Build history of the part. All positions in model axes, mm. A direction names the side the tool comes from. Round coordinates to 2 decimals unless told otherwise and drop trailing zeros. Write each loop counter-clockwise with the first axis right and the second up, starting at its lowest first coordinate (ties: lowest second). Pieces come first, ordered by that corner, then holes. Notation, with made-up numbers: (-1.5, -7) -> (11.5, -7) arc R18 ccw to (11.5, -1) -> close; hole circle Ø2 at (53, -9.5). An arc over 180 degrees is marked (long way). Answer as CSV lines item,"result".
from build123d import *

# Parameters (mm, degrees)
SKETCH_W        = 200
SKETCH_H        = 120
PAD_DEPTH       = 60
SKETCH002_R     = 16
POCKET001_DEPTH = 5
POCKET_DEPTH    = 58
SKETCH004_R     = 1.65
HOLE_DEPTH      = 4
SKETCH005_R     = 4
POCKET002_DEPTH = 3
SKETCH006_R     = 4.4
HOLE001_DEPTH   = 22.356213
HOLE001_TIPS_R  = 4.4
SKETCH007_R     = 2.5
HOLE002_DEPTH   = 25
FILLET_R        = 4.5
FILLET001_R     = 4.5
SKETCH008_R     = 1.65
HOLE003_DEPTH   = 9.00858
HOLE003_TIPS_R  = 1.65


with BuildPart() as part:
    # Sketch → Pad (new body)
    with BuildSketch(Plane.XY):
        Rectangle(SKETCH_W, SKETCH_H)
    extrude(amount=PAD_DEPTH)

    # Sketch002 (on Face3 of Pad) → Pocket001 (cut)
    with BuildSketch(Plane.XZ.offset(60)):
        with Locations((-53.5, 31)):
            Circle(SKETCH002_R)
        with Locations((-12, 31)):
            Circle(SKETCH002_R)
        with Locations((29.5, 31)):
            Circle(SKETCH002_R)
        with Locations((71, 31)):
            Circle(SKETCH002_R)
    extrude(amount=-POCKET001_DEPTH, mode=Mode.SUBTRACT)

    # Sketch003 (on Face6 of Pad) → Pocket (cut)
    with BuildSketch(Plane.XY.offset(60)):
        Polygon((-87.5, 57), (87.5, 57), (87.5, 38.5), (95.5, 38.5), (95.5, -38.5), (87.5, -38.5), (87.5, -57), (-87.5, -57), (-87.5, -38.5), (-95.5, -38.5), (-95.5, 38.5), (-87.5, 38.5), align=None)
    extrude(amount=-POCKET_DEPTH, mode=Mode.SUBTRACT)

    # Sketch004 (on Face1 of Pocket) → Hole (cut)
    with BuildSketch(Plane(origin=(0, 60, 0), x_dir=(-1, 0, 0), z_dir=(0, 1, 0))):
        with Locations((-75, 43.5)):
            Circle(SKETCH004_R)
        with Locations((12, 43.5)):
            Circle(SKETCH004_R)
        with Locations((12, 16.5)):
            Circle(SKETCH004_R)
        with Locations((-75, 16.5)):
            Circle(SKETCH004_R)
    extrude(amount=-HOLE_DEPTH, mode=Mode.SUBTRACT)

    # Sketch005 (on Face1 of Hole) → Pocket002 (cut)
    with BuildSketch(Plane(origin=(0, 60, 0), x_dir=(-1, 0, 0), z_dir=(0, 1, 0))):
        with Locations((60, 30)):
            Circle(SKETCH005_R)
    extrude(amount=-POCKET002_DEPTH, mode=Mode.SUBTRACT)

    # Sketch006 (on Face11 of Pocket002) → Hole001 (cut)
    with BuildSketch(Plane.XZ.offset(60)):
        with Locations((-78, 50)):
            Circle(SKETCH006_R)
    extrude(amount=-HOLE001_DEPTH, mode=Mode.SUBTRACT)

    # Hole001 tips → Hole001 tip 1 section 0
    with BuildSketch(Plane.XZ.offset(37.643787), mode=Mode.PRIVATE) as hole001_tip_1_s0:
        with Locations((-78, 50)):
            Circle(HOLE001_TIPS_R)
    loft([hole001_tip_1_s0.sketch, Vertex(-78, -35, 50)], mode=Mode.SUBTRACT)

    # Sketch007 (on Face11 of Hole001) → Hole002 (cut)
    with BuildSketch(Plane.XZ.offset(60)):
        with Locations((-69.5, 10)):
            Circle(SKETCH007_R)
        with Locations((-28, 10)):
            Circle(SKETCH007_R)
        with Locations((13.5, 10)):
            Circle(SKETCH007_R)
        with Locations((55, 10)):
            Circle(SKETCH007_R)
    extrude(amount=-HOLE002_DEPTH, mode=Mode.SUBTRACT)

    # Fillet
    fillet_edges = [part.edges().sort_by_distance(p)[0] for p in [
        (-100, -60, 30),
        (-100, 60, 30),
        (100, -60, 30),
        (100, 60, 30),
    ]]
    fillet(fillet_edges, radius=FILLET_R)

    # Fillet001
    fillet001_edges = [part.edges().sort_by_distance(p)[0] for p in [
        (87.5, 38.5, 31),
        (-87.5, 38.5, 31),
        (-87.5, -38.5, 31),
        (87.5, -38.5, 31),
    ]]
    fillet(fillet001_edges, radius=FILLET001_R)

    # Sketch008 (on Face11 of Hole002) → Hole003 (cut)
    with BuildSketch(Plane.XZ.offset(60)):
        with Locations((-53.5, 55.25)):
            Circle(SKETCH008_R)
        with Locations((-12, 55.25)):
            Circle(SKETCH008_R)
        with Locations((29.5, 55.25)):
            Circle(SKETCH008_R)
        with Locations((71, 55.25)):
            Circle(SKETCH008_R)
        with Locations((71, 6.75)):
            Circle(SKETCH008_R)
        with Locations((29.5, 6.75)):
            Circle(SKETCH008_R)
        with Locations((-12, 6.75)):
            Circle(SKETCH008_R)
        with Locations((-53.5, 6.75)):
            Circle(SKETCH008_R)
    extrude(amount=-HOLE003_DEPTH, mode=Mode.SUBTRACT)

    # Hole003 tips → Hole003 tip 1 section 0
    with BuildSketch(Plane.XZ.offset(50.99142), mode=Mode.PRIVATE) as hole003_tip_1_s0:
        with Locations((-53.5, 55.25)):
            Circle(HOLE003_TIPS_R)
    loft([hole003_tip_1_s0.sketch, Vertex(-53.5, -50, 55.25)], mode=Mode.SUBTRACT)

    # Hole003 tips → Hole003 tip 2 section 0
    with BuildSketch(Plane.XZ.offset(50.99142), mode=Mode.PRIVATE) as hole003_tip_2_s0:
        with Locations((-12, 55.25)):
            Circle(HOLE003_TIPS_R)
    loft([hole003_tip_2_s0.sketch, Vertex(-12, -50, 55.25)], mode=Mode.SUBTRACT)

    # Hole003 tips → Hole003 tip 3 section 0
    with BuildSketch(Plane.XZ.offset(50.99142), mode=Mode.PRIVATE) as hole003_tip_3_s0:
        with Locations((29.5, 55.25)):
            Circle(HOLE003_TIPS_R)
    loft([hole003_tip_3_s0.sketch, Vertex(29.5, -50, 55.25)], mode=Mode.SUBTRACT)

    # Hole003 tips → Hole003 tip 4 section 0
    with BuildSketch(Plane.XZ.offset(50.99142), mode=Mode.PRIVATE) as hole003_tip_4_s0:
        with Locations((71, 55.25)):
            Circle(HOLE003_TIPS_R)
    loft([hole003_tip_4_s0.sketch, Vertex(71, -50, 55.25)], mode=Mode.SUBTRACT)

    # Hole003 tips → Hole003 tip 5 section 0
    with BuildSketch(Plane.XZ.offset(50.99142), mode=Mode.PRIVATE) as hole003_tip_5_s0:
        with Locations((71, 6.75)):
            Circle(HOLE003_TIPS_R)
    loft([hole003_tip_5_s0.sketch, Vertex(71, -50, 6.75)], mode=Mode.SUBTRACT)

    # Hole003 tips → Hole003 tip 6 section 0
    with BuildSketch(Plane.XZ.offset(50.99142), mode=Mode.PRIVATE) as hole003_tip_6_s0:
        with Locations((29.5, 6.75)):
            Circle(HOLE003_TIPS_R)
    loft([hole003_tip_6_s0.sketch, Vertex(29.5, -50, 6.75)], mode=Mode.SUBTRACT)

    # Hole003 tips → Hole003 tip 7 section 0
    with BuildSketch(Plane.XZ.offset(50.99142), mode=Mode.PRIVATE) as hole003_tip_7_s0:
        with Locations((-12, 6.75)):
            Circle(HOLE003_TIPS_R)
    loft([hole003_tip_7_s0.sketch, Vertex(-12, -50, 6.75)], mode=Mode.SUBTRACT)

    # Hole003 tips → Hole003 tip 8 section 0
    with BuildSketch(Plane.XZ.offset(50.99142), mode=Mode.PRIVATE) as hole003_tip_8_s0:
        with Locations((-53.5, 6.75)):
            Circle(HOLE003_TIPS_R)
    loft([hole003_tip_8_s0.sketch, Vertex(-53.5, -50, 6.75)], mode=Mode.SUBTRACT)


solid = part.part
1. Mould opens along Z. For faces 4 (the flat face through (-87.5, -50, 31)), 5 (the flat face through (1, 1, 2)), 6 (the cylindrical face through (26.03, -58.52, 15.38)) say: +Z half, -Z half, draft (parallel to the pull), parting line (faces both ways), or undercut.
Results found:
face 4,"draft"
face 5,"+Z half"
face 6,"undercut"
2. Cut at B-B, the plane y = -7.5. Write the cut outline in (x, z).
Results found:
outline,"(-100, 0) -> (100, 0) -> (100, 60) -> (95.5, 60) -> (95.5, 2) -> (-95.5, 2) -> (-95.5, 60) -> (-100, 60) -> close"
3. Cut at D-D, the plane z = 39.5. Count the separate pieces of the cut face and the enclosed holes in it, then the cut area to 3 significant figures.
Results found:
separate pieces,"4"
enclosed holes,"0"
area,"2,460 mm2"
4. Drop flat-ended pins along their axis: pin 1 Ø5.5 at (x, z) = (71, 6.75) entering from -Y; pin 2 Ø19 at (x, z) = (71, 31) entering from -Y; pin 3 Ø3 at (x, z) = (-12, 43.5) entering from +Y. Give the stop position or say it passes through.
Results found:
pin 1,"stops at y = -60"
pin 2,"stops at y = 57"
pin 3,"passes through"
5. Probe line 1 along Z through (x, y) = (-12, -58.05); line 2 along Z through (x, y) = (-12, 57.8); line 3 along X through (y, z) = (-29, 28). List the from-to ranges inside material, lowest first.
Results found:
line 1,"z = 0 to 5.1, 8.4 to 15, 47 to 53.6, 56.9 to 60"
line 2,"z = 0 to 14.85, 18.15 to 41.85, 45.15 to 60"
line 3,"x = -100 to -95.5, 95.5 to 100"
6. Cut at C-C, the plane x = 49.5. Write the cut outline in (y, z).
Results found:
outline,"(-60, 0) -> (60, 0) -> (60, 60) -> (57, 60) -> (57, 2) -> (-57, 2) -> (-57, 60) -> (-60, 60) -> close"
7. Cut at A-A, the plane x = -78. Write the cut outline in (y, z), then the cut area to 3 significant figures.
Results found:
outline,"(-60, 0) -> (60, 0) -> (60, 60) -> (57, 60) -> (57, 2) -> (-57, 2) -> (-57, 45.6) -> (-60, 45.6) -> close; (-60, 54.4) -> (-57, 54.4) -> (-57, 60) -> (-60, 60) -> close"
area,"562 mm2"
8. Which spindle directions (+Z, -Z, +X, -X, +Y, -Y) get a long thin tool onto all of the face, cutting with end or side? Do faces 1 (the cylindrical face through (-66.197, -58.521, 21.264)), 2 (the flat face through (-87.5, 50, 31)), 3 (the cylindrical face through (-63.815, 58.521, 31.201)). Say none if no direction does.
Results found:
face 1,"-Y"
face 2,"+Z"
face 3,"+Y, -Y"
